from build123d import *

# Parameters (mm, degrees)
F0_W      = 111
F0_H      = 20
F1_DEPTH  = 150
F2_R      = 14.996
F3_DEPTH  = 35
F4_R      = 14.996
F4_R_2    = 13.4495
F5_DEPTH  = 3
F6_R      = 14.996
F6_R_2    = 13.4495
F7_DEPTH  = 1.22
F8_R      = 16.996
F9_DEPTH  = 4
F10_R     = 8.540661
F11_DEPTH = 2
F12_R     = 5
F13_DEPTH = 20.001
F14_R     = 3
F15_DEPTH = 26.001
F16_R     = 5.6
F17_DEPTH = 16


with BuildPart() as f1:
    # F0 (on Front) → F1 (new body)
    with BuildSketch(Plane.XZ):
        with Locations((0.662768, -21.843081)):
            Rectangle(F0_W, F0_H)
    extrude(amount=F1_DEPTH)

    # F2 (on face) → F3 (join)
    with BuildSketch(Plane.XY.offset(-11.843081)):
        with Locations((0.662768, -85.246)):
            Circle(F2_R)
        with BuildLine():
            ThreePointArc((6.768928, -87.025451), (-5.697392, -85.246), (6.768928, -83.466549))
            Line((6.768928, -83.466549), (6.768928, -87.025451))
        make_face(mode=Mode.SUBTRACT)
    extrude(amount=F3_DEPTH)

    # F4 (on face) → F5 (cut)
    with BuildSketch(Plane.XY.offset(23.156919)):
        with Locations((0.662768, -85.246)):
            Circle(F4_R)
        with Locations((0.662768, -85.246)):
            Circle(F4_R_2, mode=Mode.SUBTRACT)
    extrude(amount=-F5_DEPTH, mode=Mode.SUBTRACT)

    # F6 (on face) → F7 (join)
    with BuildSketch(Plane.XY.offset(23.156919)):
        with Locations((0.662768, -85.246)):
            Circle(F6_R)
        with Locations((0.662768, -85.246)):
            Circle(F6_R_2, mode=Mode.SUBTRACT)
    extrude(amount=-F7_DEPTH)

    # F8 (on face) → F9 (join)
    with BuildSketch(Plane.XY.offset(-11.843081)):
        with Locations((0.662768, -85.246)):
            Circle(F8_R)
    extrude(amount=F9_DEPTH)

    # F10 (on face) → F11 (join)
    with BuildSketch(Plane.XY.offset(-7.843081)):
        with Locations((0.662768, -85.246)):
            Circle(F10_R)
    extrude(amount=F11_DEPTH)

    # F12 (on face) → F13 (cut, through all)
    with BuildSketch(Plane.XY.offset(-11.843081)):
        with Locations((36.962768, -16.625)):
            Circle(F12_R)
        with Locations((12.762768, -16.625)):
            Circle(F12_R)
        with Locations((-11.437232, -16.625)):
            Circle(F12_R)
        with Locations((-35.637232, -16.625)):
            Circle(F12_R)
    extrude(amount=-F13_DEPTH, mode=Mode.SUBTRACT)

    # F14 (on face) → F15 (cut, through all)
    with BuildSketch(Plane.XY.offset(-5.843081)):
        with Locations((0.662768, -85.246)):
            Circle(F14_R)
    extrude(amount=-F15_DEPTH, mode=Mode.SUBTRACT)

    # F16 (on face) → F17 (cut)
    with BuildSketch(Plane(origin=(0, 0, -31.843081), x_dir=(1, 0, 0), z_dir=(0, 0, -1))):
        with Locations((0.662768, 85.246)):
            Circle(F16_R)
    extrude(amount=-F17_DEPTH, mode=Mode.SUBTRACT)


solid = f1.part
Here's how the part is built. I have some questions about the finished solid (model axes, mm). A direction names the side the tool comes from. Round coordinates to 2 decimals unless told otherwise and drop trailing zeros. Order: outer loops, then holes, each group sorted by start corner. A loop starts at its lowest first (then second) coordinate and runs counter-clockwise, first axis right, second up. Notation, with made-up numbers: M 28.25,60 L 37.25,60 A34 cw 37.25,95 Z; hole C -34.5,37.25 d2. An arc over 180 degrees is marked long. Return JSON: item names as keys, results as strings. Group by question number.
1. I'm going to push flat-ended pins straight in: pin 1 Ø12 at (y, z) = (-74, 11.5) entering from -X; pin 2 Ø6 at (x, z) = (9, 11.5) entering from -Y; pin 3 Ø6 at (x, y) = (3, -87.5) entering from +Z. Where does each tip first touch, or does it pass through?
2. If we section it at C-C on y = -47: List the corners of the cut face in (x, z) for me.
3. On a 3-axis mill with a long thin cutter (end or side, diameter ignored), from which of +Z, -Z, +X, -X, +Y, -Y can I reach the whole of each face in a straight line? I mean faces 1 (the face through (-54.837, -74, -22)), 2 (the face through (2, -82, -5.843)), 3 (the face through (-1.6, -71.8, 20.157)), 4 (the face through (3.25, -80.28, -23.96)). Say none if no direction works.
4. If we mould it in two halves opening along X, with no side actions, what happens to faces 5 (the face through (3, -83, -15.843)), 6 (the face through (56.163, -74, -22)), 7 (the face through (7.58, -98.55, 22.56))? For each: pulls with the +X half, pulls with the -X half, needs draft (parallel to the pull), parting line crosses it, or undercut.
5. If we section it at D-D on x = -24: List the corners of the cut face in (y, z) for me.
6. If we section it at A-A on x = 11: List the corners of the cut face in (y, z) for me.
7. If we section it at B-B on z = -2: List the corners of the cut face in (x, y) for me.
8. Please list where these lines run through material, in increasing order: probe 1 along Z at (x, y) = (17.5, -133.5); probe 2 along X at (y, z) = (-12.5, -27); probe 3 along Y at (x, z) = (7.5, 5).
Reply:
{
 "1": {"pin 1": "x = -13.39", "pin 2": "y = -99.26", "pin 3": "z = -5.84"},
 "2": {"outline": "M -54.84,-31.84 L 56.16,-31.84 L 56.16,-11.84 L -54.84,-11.84 Z"},
 "3": {"face 1": "+Z, -Z, -X, +Y, -Y", "face 2": "+Z", "face 3": "none", "face 4": "-Z"},
 "4": {"face 5": "undercut", "face 6": "pulls with the +X half", "face 7": "parting line crosses it"},
 "5": {"outline": "M -150,-31.84 L 0,-31.84 L 0,-11.84 L -150,-11.84 Z"},
 "6": {"outline": "M -150,-31.84 L -21.3,-31.84 L -21.3,-11.84 L -71.76,-11.84 L -71.76,-7.84 L -74.38,-7.84 L -74.38,20.16 L -76.64,20.16 L -76.64,21.94 L -74.38,21.94 L -74.38,23.16 L -96.11,23.16 L -96.11,21.94 L -93.85,21.94 L -93.85,20.16 L -96.11,20.16 L -96.11,-7.84 L -98.74,-7.84 L -98.74,-11.84 L -150,-11.84 Z; M -11.95,-31.84 L 0,-31.84 L 0,-11.84 L -11.95,-11.84 Z"},
 "7": {"outline": "C 0.66,-85.25 d29.99; hole M 6.77,-87.03 L 6.77,-83.47 A6.36 ccw long Z"},
 "8": {"probe 1": "-31.84 to -11.84", "probe 2": "-54.84 to -38.46, -32.81 to -14.26, -8.61 to 9.94, 15.59 to 34.14, 39.79 to 56.16", "probe 3": "-98.59 to -71.9"}
}
